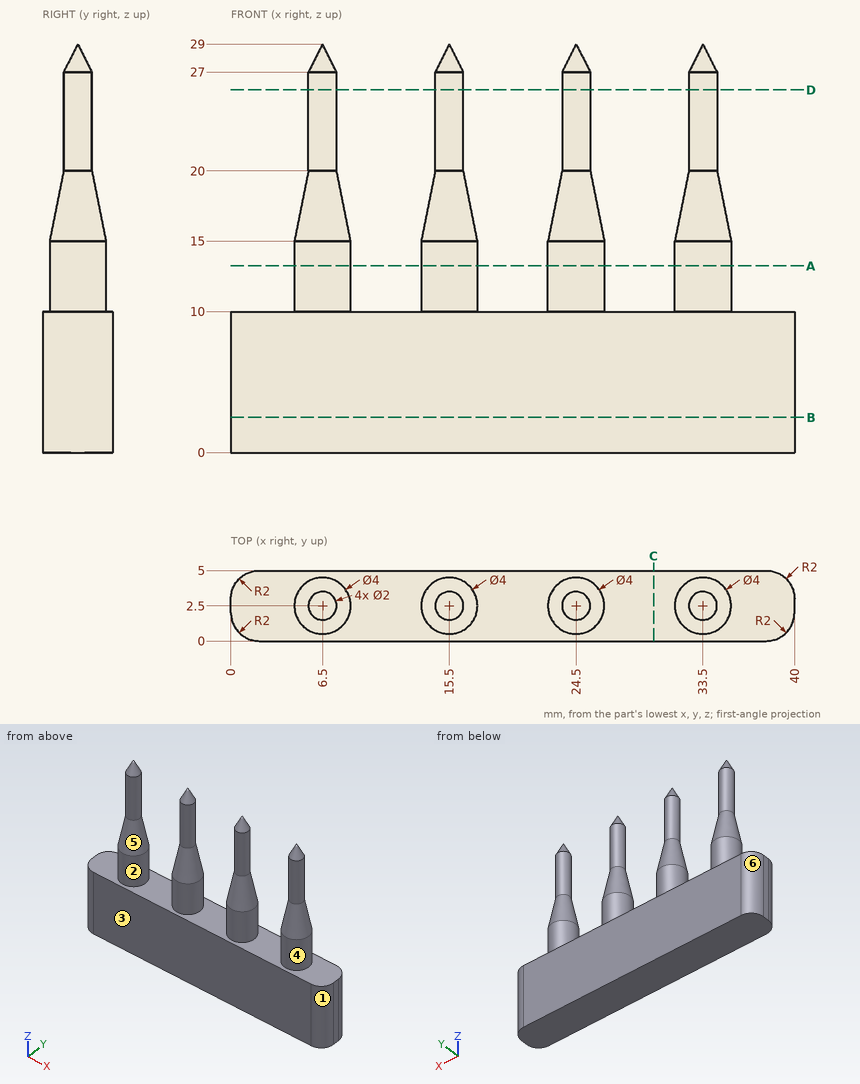
Design review of the part shown in the three views and the two pictorial views. Dimensions are in mm from the part's minimum x, y and z. A direction names the side the tool comes from. Give positions to 0.01 mm unless a question says otherwise; leave off trailing zeros. Loops run counter-clockwise (first coordinate to the right, second up) from the corner with the lowest first, then second, coordinate; pieces in that order, holes last. Notation, with made-up numbers: M 2.5,-20.75 L 38.5,-20.75 A18 cw 38.5,-10.75 Z; hole C 25.25,3.25 d10. An arc over 180 degrees is marked long. Answer as a JSON object with one key per item and string values. Group by question number.
Q1. Add section C-C on x = 30. Give the boundary of the cut face in (y, z).
Q2. Add section A-A on z = 13.25. Give the boundary of the cut face in (x, y), and give its area (3 significant figures).
Q3. Insertion check: P1, Ø3, axis at y = 3, z = 22, coming from the -X side; P2, Ø3, axis at x = 31.5, z = 17.5, coming from the +Y side; P3, Ø2.5, axis at x = 11, y = 3.5, coming from the +Z side. Each pin has a flat end and moves straight along its axis. Give the tip position at first contact, or say it passes through.
Q4. For probe 1 along X at (y, z) = (1.7, 18.75); probe 2 along X at (y, z) = (1.1, 12.5); probe 3 along Z at (x, y) = (17.5, 1.55), list the stretches that pass through material, from the lowest coordinate up. Write a range as [from, to].
Q5. Tool access review of the marked faces 1 and 2: name each direction out of +Z, -Z, +X, -X, +Y, -Y from which nothing blocks a thin tool from reaching the whole face with its end or side.
Q6. Add section D-D on z = 25.75. Give the boundary of the cut face in (x, y), and give its area (3 significant figures).
Q7. Mouldability with a two-part tool opening along X and no side actions: class the marked faces 3, 4, 5 and 6 as +X half, -X half, draft (parallel to the pull), parting line (faces both ways), or undercut.
Q8. Add section B-B on z = 2.5. Give the boundary of the cut face in (x, y), and give its area (3 significant figures).
Checked values:
{
 "1": {"outline": "M 0,0 L 5,0 L 5,10 L 0,10 Z"},
 "2": {"outline": "C 6.5,2.5 d4; C 15.5,2.5 d4; C 24.5,2.5 d4; C 33.5,2.5 d4", "area": "50.3 mm²"},
 "3": {"P1": "x = 5.5", "P2": "y = 4", "P3": "z = 10"},
 "4": {"probe 1": "[5.54, 7.46], [14.54, 16.46], [23.54, 25.46], [32.54, 34.46]", "probe 2": "[5.07, 7.93], [14.07, 16.93], [23.07, 25.93], [32.07, 34.93]", "probe 3": "[0, 10]"},
 "5": {"face 1": "+Z, -Z, +X, -Y", "face 2": "+Z"},
 "6": {"outline": "C 6.5,2.5 d2; C 15.5,2.5 d2; C 24.5,2.5 d2; C 33.5,2.5 d2", "area": "12.6 mm²"},
 "7": {"face 3": "draft", "face 4": "undercut", "face 5": "undercut", "face 6": "-X half"},
 "8": {"outline": "M 0,2 A2 ccw 2,0 L 38,0 A2 ccw 40,2 L 40,3 A2 ccw 38,5 L 2,5 A2 ccw 0,3 Z", "area": "197 mm²"}
}
